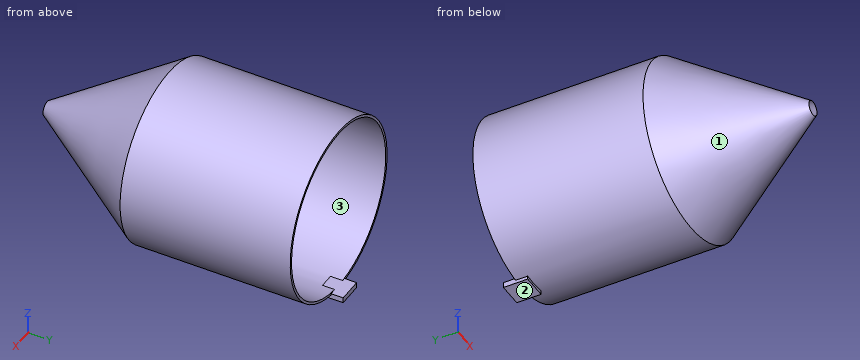
```python
from build123d import *

# Parameters (mm, degrees)
SKETCH2_R           = 2
SKETCH2_R_2         = 5
CUT_EXTRUDE1_DEPTH  = 3
SKETCH3_W           = 10
SKETCH3_H           = 2.237585103
BOSS_EXTRUDE1_DEPTH = 5


with BuildPart() as part:
    # Sketch1 → Revolve1 (revolve)
    with BuildSketch(Plane.XY, mode=Mode.PRIVATE) as revolve1_sk:
        Polygon((2.310834394, 103.017979097), (2.310834394, 34.01998915), (-32.689165606, 34.01998915), (-32.689165606, 33.01998915), (2.310836414, 33.01998915), (-29.686396209, -16.982020903), (3.310834394, 33.017979097), (3.310834394, 103.017979097), align=None)
    revolve(revolve1_sk.sketch.rotate(Axis((-32.689165606, 34.01998915, 0), (0, -1, 0)), 90), axis=Axis((-32.689165606, 34.01998915, 0), (0, -1, 0)))

    # Sketch2 → Cut-Extrude1 (cut)
    with BuildSketch(Plane(origin=(0, 34.01998915, 0), x_dir=(1, 0, 0), z_dir=(0, 1, 0))):
        with Locations(Location((-32.689165606, 0, 0), (0, 0, 270))):
            Circle(SKETCH2_R)
        with Locations(Location((-14.583845408, 17.239413579, 0), (0, 0, 270))):
            Circle(SKETCH2_R_2)
    extrude(amount=-CUT_EXTRUDE1_DEPTH, mode=Mode.SUBTRACT)

    # Sketch3 → Boss-Extrude1 (add, symmetric)
    with BuildSketch(Plane(origin=(0, 103.017979097, 0), x_dir=(1, 0, 0), z_dir=(0, 1, 0))):
        with Locations((-32.016176603, 35.993708975)):
            Rectangle(SKETCH3_W, SKETCH3_H)
    extrude(amount=BOSS_EXTRUDE1_DEPTH, both=True)


solid = part.part
```
The listing builds one solid part. Answer for the finished solid, in the listing's coordinates (mm). Face numbers are marked on the shaded views. Round coordinates to 2 decimals unless told otherwise and drop trailing zeros. Order: outer loops, then holes, each group sorted by start corner. A loop starts at its lowest first (then second) coordinate and runs counter-clockwise, first axis right, second up. Notation, with made-up numbers: (-26, -10.5) - (15, -10.5) arc R11 ccw to (15, 4.5) - close; hole circle Ø2 at (-36, -31.5). An arc over 180 degrees is marked (long way). Put each result on its own line as item: value. Start each with the question number.
(1) Find section C-C (y = 9). Give the vertices of the cut face in (x, z), plus the area to 3 significant figures.
(2) Given P1, Ø2.5, axis at y = 104.5, z = -36.5, coming from the +X side; P2, Ø2, axis at x = -22.5, y = 6.5, coming from the +Z side; P3, Ø6, axis at x = -26, z = -19, coming from the +Y side; P4, Ø4, axis at x = -33.5, z = 2, coming from the -Y side, each flat-ended and moving along its own axis, determine where each tip first touches the part or whether it passes through.
(3) Determine the mould class of the marked faces 1, 2 and 3 for opening direction Z: released by +Z, released by -Z, zero draft, split by the parting line, or undercut.
(4) Straight lines are drawn through the part: probe 1 along X at (y, z) = (67, 0); probe 2 along X at (y, z) = (33.85, 0); probe 3 along Z at (x, y) = (-37, -2.5). For each, find the intervals that lie inside material, in ascending order. Write a range as from..to.
(5) Find section B-B (y = 79). Give the vertices of the cut face in (x, z), plus the area to 3 significant figures.
(6) Find section A-A (z = 0). Give the vertices of the cut face in (x, y).
Reply:
1. outline: circle Ø40.3 at (-32.69, 0); hole circle Ø39.26 at (-32.69, 0)
1. area: 65.0 mm^2
2. P1: x = -27.02
2. P2: z = 16.43
2. P3: y = 34.02
2. P4: y = -16.98
3. face 1: split by the parting line
3. face 2: released by -Z
3. face 3: undercut
4. probe 1: -68.69..-67.69, 2.31..3.31
4. probe 2: -68.69..-34.69, -30.69..3.31
4. probe 3: -11.8..-11.49, 11.49..11.8
5. outline: circle Ø72 at (-32.69, 0); hole circle Ø70 at (-32.69, 0)
5. area: 223 mm^2
6. outline: (-68.69, 33.02) - (-35.69, -16.98) - (-67.69, 33.02) - (-34.69, 33.02) - (-34.69, 34.02) - (-67.69, 34.02) - (-67.69, 103.02) - (-68.69, 103.02) - close; (-30.69, 33.02) - (2.31, 33.02) - (-29.69, -16.98) - (3.31, 33.02) - (3.31, 103.02) - (2.31, 103.02) - (2.31, 34.02) - (-30.69, 34.02) - close
